```python
from build123d import *

# Parameters (mm, degrees)
SKETCH_1_R      = 1.65
EXTRUDE_1_DEPTH = 8
FILLET_1_R      = 3


with BuildPart() as part:
    # 草图1 → 凸台-拉伸1 (new body)
    with BuildSketch(Plane(origin=(0, 0, 0), x_dir=(1, 0, 0), z_dir=(0, 1, 0))):
        with BuildLine():
            Line((-19, 12.5), (-19, -12.5))
            ThreePointArc((-19, -12.5), (-17.828427125, -15.328427125), (-15, -16.5))
            Line((-15, -16.5), (15, -16.5))
            ThreePointArc((15, -16.5), (17.828427125, -15.328427125), (19, -12.5))
            Line((19, -12.5), (19, 12.5))
            ThreePointArc((19, 12.5), (17.828427125, 15.328427125), (15, 16.5))
            Line((15, 16.5), (-15, 16.5))
            ThreePointArc((-15, 16.5), (-17.828427125, 15.328427125), (-19, 12.5))
        make_face()
        with Locations(Location((-15, 12.5, 0), (0, 0, 270))):
            Circle(SKETCH_1_R, mode=Mode.SUBTRACT)
        with Locations(Location((15, 12.5, 0), (0, 0, 270))):
            Circle(SKETCH_1_R, mode=Mode.SUBTRACT)
        with Locations(Location((-15, -12.5, 0), (0, 0, 270))):
            Circle(SKETCH_1_R, mode=Mode.SUBTRACT)
        with Locations(Location((15, -12.5, 0), (0, 0, 270))):
            Circle(SKETCH_1_R, mode=Mode.SUBTRACT)
        with BuildLine():
            Line((-11, 12.5), (11, 12.5))
            ThreePointArc((11, 12.5), (12.171572875, 9.671572875), (15, 8.5))
            Line((15, 8.5), (15, -8.5))
            ThreePointArc((15, -8.5), (12.171572875, -9.671572875), (11, -12.5))
            Line((11, -12.5), (-11, -12.5))
            ThreePointArc((-11, -12.5), (-12.171572875, -9.671572875), (-15, -8.5))
            Line((-15, -8.5), (-15, 8.5))
            ThreePointArc((-15, 8.5), (-12.171572875, 9.671572875), (-11, 12.5))
        make_face(mode=Mode.SUBTRACT)
    extrude(amount=EXTRUDE_1_DEPTH)

    # 圆角1
    fillet_1_edges = [part.edges().sort_by_distance(p)[0] for p in [
        (-11, 4, -12.5),
        (-15, 4, -8.5),
        (-15, 4, 8.5),
        (-11, 4, 12.5),
        (11, 4, 12.5),
        (15, 4, 8.5),
        (15, 4, -8.5),
        (11, 4, -12.5),
    ]]
    fillet(fillet_1_edges, radius=FILLET_1_R)


solid = part.part
```
CAD build for the part. Positions are in the model's coordinates, mm. A direction names the side the tool comes from. Round coordinates to 2 decimals unless told otherwise and drop trailing zeros. Order: outer loops, then holes, each group sorted by start corner. A loop starts at its lowest first (then second) coordinate and runs counter-clockwise, first axis right, second up. Notation, with made-up numbers: (82.5, -28.5) - (121.5, -28.5) arc R15 cw to (121.5, -14.5) - close; hole circle Ø11 at (-25.5, 42.5). An arc over 180 degrees is marked (long way). Use CSV: the item, a comma, the result in double quotes. Start each with the question number.
1) Pin check, flat tip, straight feed: pin 1 Ø2 at (x, z) = (11.5, 7.5) entering from -Y. Stop position of the tip, or through.
2) Saw through at C-C (x = 3). List the corners of the cut face in (y, z).
3) Wall check: L1, parallel to Z at x = -4, y = 4; L2, parallel to X at y = 3.25, z = 6; L3, parallel to Z at x = -11, y = 2.25. Give the ranges that are in metal, low to high. Write a range as [from, to].
4) Saw through at A-A (z = 2). List the corners of the cut face in (x, y), and give its area (3 significant figures).
5) Saw through at B-B (y = 7.5). List the corners of the cut face in (x, z), and give its area (3 significant figures).
6) Tool access for faces 1 (the flat face through (-15, 4, 0)), 2 (the flat face through (0, 0, -15)): list every direction of +Z, -Z, +X, -X, +Y, -Y with a clear straight run to the whole face (end or side of a thin tool).
7) Saw through at D-D (z = -12). List the corners of the cut face in (x, y).
8) Two-plate mould, pull along Z, no slides. Class faces 3 (the cylindrical face through (-17.859, 3.944, 15.297)), 4 (the flat face through (-19, 4, 0)), 5 (the cylindrical face through (14.548, 4.056, -7.759)), 6 (the cylindrical face through (12.158, 3.944, -9.685)): pulls with the +Z half, pulls with the -Z half, needs draft (parallel to the pull), parting line crosses it, or undercut.
Values follow:
1,pin 1,"passes through"
2,outline,"(0, -16.5) - (8, -16.5) - (8, -12.5) - (0, -12.5) - close; (0, 12.5) - (8, 12.5) - (8, 16.5) - (0, 16.5) - close"
3,L1,"z = [-16.5, -12.5], [12.5, 16.5]"
3,L2,"x = [-19, -15], [15, 19]"
3,L3,"z = [-16.5, -11.4], [11.4, 16.5]"
4,outline,"(-19, 0) - (-15, 0) - (-15, 8) - (-19, 8) - close; (15, 0) - (19, 0) - (19, 8) - (15, 8) - close"
4,area,"64.0 mm2"
5,outline,"(-19, -12.5) arc R4 ccw to (-15, -16.5) - (15, -16.5) arc R4 ccw to (19, -12.5) - (19, 12.5) arc R4 ccw to (15, 16.5) - (-15, 16.5) arc R4 ccw to (-19, 12.5) - close; hole circle Ø3.3 at (-15, -12.5); hole circle Ø3.3 at (-15, 12.5); hole (-15, -6.18) arc R3 ccw to (-13.29, -8.89) arc R4 cw to (-11.39, -10.79) arc R3 ccw to (-8.68, -12.5) - (8.68, -12.5) arc R3 ccw to (11.39, -10.79) arc R4 cw to (13.29, -8.89) arc R3 ccw to (15, -6.18) - (15, 6.18) arc R3 ccw to (13.29, 8.89) arc R4 cw to (11.39, 10.79) arc R3 ccw to (8.68, 12.5) - (-8.68, 12.5) arc R3 ccw to (-11.39, 10.79) arc R4 cw to (-13.29, 8.89) arc R3 ccw to (-15, 6.18) - close; hole circle Ø3.3 at (15, -12.5); hole circle Ø3.3 at (15, 12.5)"
5,area,"513 mm2"
6,face 1,"+Y, -Y"
6,face 2,"+Z, -Z, +X, -X, -Y"
7,outline,"(-19, 0) - (-16.57, 0) - (-16.57, 8) - (-19, 8) - close; (-13.43, 0) - (-10.33, 0) - (-10.33, 8) - (-13.43, 8) - close; (10.33, 0) - (13.43, 0) - (13.43, 8) - (10.33, 8) - close; (16.57, 0) - (19, 0) - (19, 8) - (16.57, 8) - close"
8,face 3,"pulls with the +Z half"
8,face 4,"needs draft"
8,face 5,"undercut"
8,face 6,"undercut"
